For this review, use the dimensioned drawing (mm, ordinates from the lowest corner) and the shaded views. Round coordinates to 2 decimals unless told otherwise and drop trailing zeros. Loops run counter-clockwise (first coordinate to the right, second up) from the corner with the lowest first, then second, coordinate; pieces in that order, holes last. Notation, with made-up numbers: (-36.5, 30) - (11.5, 30) arc R20 ccw to (11.5, 47) - close; hole circle Ø1 at (29.25, 72.5). An arc over 180 degrees is marked (long way). Use one line per item in the form item = value. Start each with the question number.
(1) Wall thickness on probe 1 along X at (y, z) = (2.65, 15); probe 2 along X at (y, z) = (1.45, 15); probe 3 along Z at (x, y) = (15, 2.5): over which ranges is each line inside the solid? List them lowest first. Write a range as [from, to].
(2) We need section D-D, the plane z = 22.5. Write out the cut boundary in (x, y), then the cut area to 3 significant figures.
(3) We need section A-A, the plane z = 15. Write out the cut boundary in (x, y), then the cut area to 3 significant figures.
(4) For pin 1 (1.5 mm diameter, centred on x = 36.5, z = 4, fed in from -Y); pin 2 (10.5 mm diameter, centred on x = 15, z = 15, fed in from -Y), all flat-tipped, find the tip position at first contact; note any pin that passes through.
(5) We need section B-B, the plane x = 38. Write out the cut boundary in (y, z), then the cut area to 3 significant figures.
(6) We need section C-C, the plane y = 0.65. Write out the cut boundary in (x, z), then the cut area to 3 significant figures.
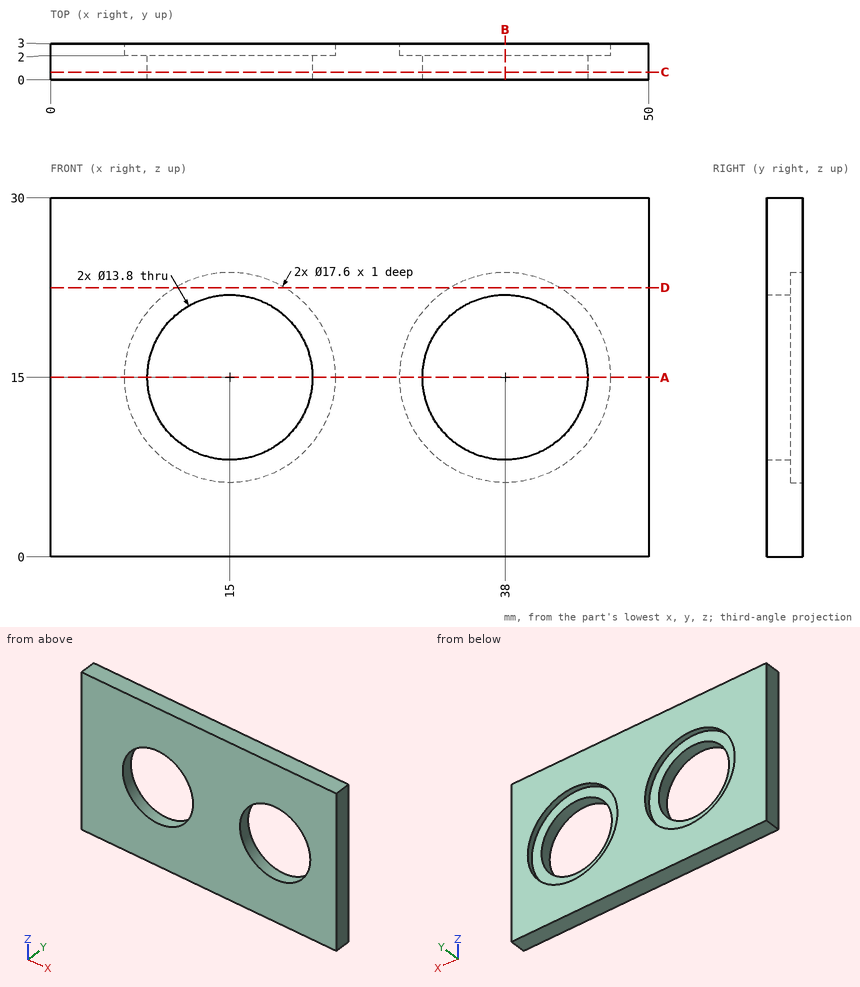
Data:
q1.probe_1 = [0, 6.2], [23.8, 29.2], [46.8, 50]
q1.probe_2 = [0, 8.1], [21.9, 31.1], [44.9, 50]
q1.probe_3 = [0, 6.2], [23.8, 30]
q2.outline = (0, 0) - (50, 0) - (50, 3) - (42.6, 3) - (42.6, 2) - (33.4, 2) - (33.4, 3) - (19.6, 3) - (19.6, 2) - (10.4, 2) - (10.4, 3) - (0, 3) - close
q2.area = 132 mm^2
q3.outline = (0, 0) - (8.1, 0) - (8.1, 2) - (6.2, 2) - (6.2, 3) - (0, 3) - close; (21.9, 0) - (31.1, 0) - (31.1, 2) - (29.2, 2) - (29.2, 3) - (23.8, 3) - (23.8, 2) - (21.9, 2) - close; (44.9, 0) - (50, 0) - (50, 3) - (46.8, 3) - (46.8, 2) - (44.9, 2) - close
q3.area = 59.6 mm^2
q4.pin_1 = 0
q4.pin_2 = through
q5.outline = (0, 0) - (3, 0) - (3, 6.2) - (2, 6.2) - (2, 8.1) - (0, 8.1) - close; (0, 21.9) - (2, 21.9) - (2, 23.8) - (3, 23.8) - (3, 30) - (0, 30) - close
q5.area = 44.8 mm^2
q6.outline = (0, 0) - (50, 0) - (50, 30) - (0, 30) - close; hole circle Ø13.8 at (15, 15); hole circle Ø13.8 at (38, 15)
q6.area = 1,200 mm^2
